Could you check a few things on this drawing? It's one solid part, dimensions in mm from its lowest x, y, z. Coordinates: 2 decimals unless noted, no trailing zeros. Write each loop counter-clockwise with the first axis right and the second up, starting at its lowest first coordinate (ties: lowest second). Pieces come first, ordered by that corner, then holes. Notation, with made-up numbers: (-33.75, 80) - (-19.75, 80) arc R20 ccw to (-19.75, 104) - close; hole circle Ø7 at (22, 41.25). An arc over 180 degrees is marked (long way). Write item = value, one per line. Start each with the question number.
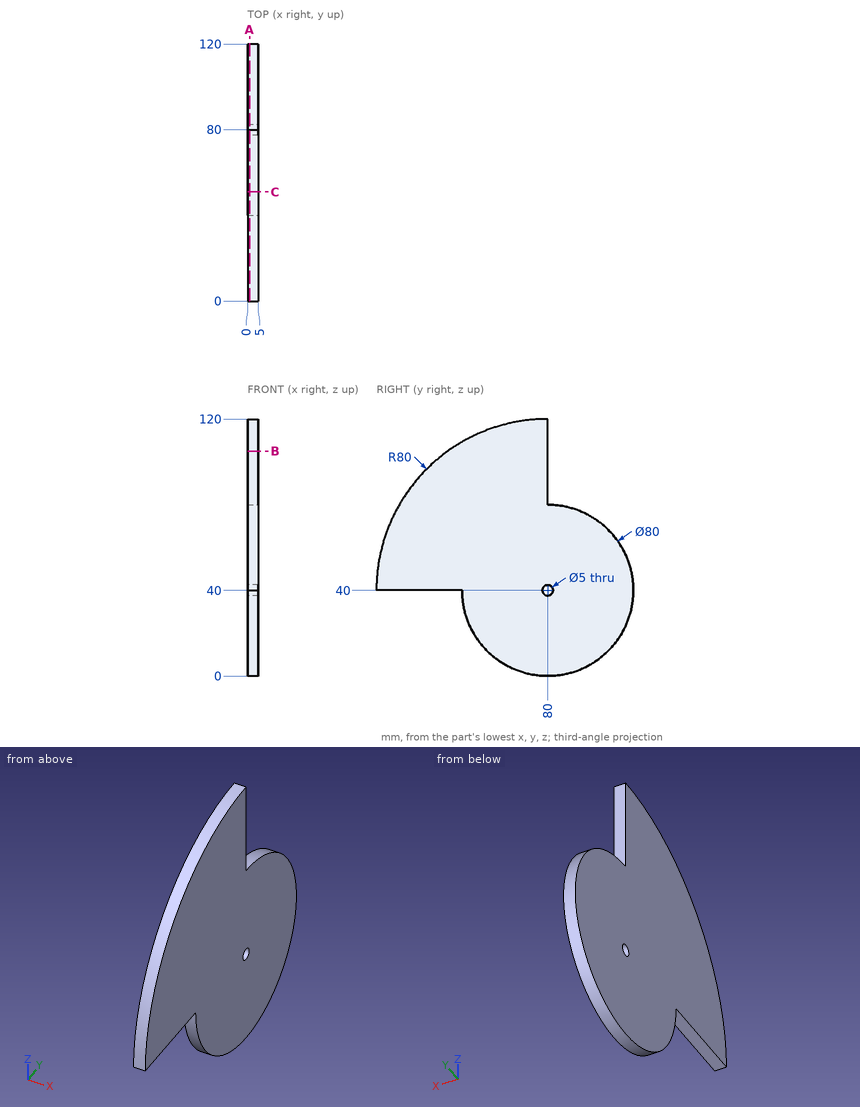
1) Suppose I cut it at B-B on z = 105. Please give me the cut outline in (x, y).
2) Suppose I cut it at A-A on x = 0.9. Please give me the cut outline in (y, z).
3) If I drill on probe 1 along Y at (x, z) = (3.35, 39); probe 2 along Y at (x, z) = (0.35, 28); probe 3 along Y at (x, z) = (3.95, 59.5), over which ranges is the centre line in solid material (lowest first)? Write a range as [from, to].
4) Suppose I cut it at C-C on y = 51. Please give me the cut outline in (x, z), plus the area to 3 significant figures.
5) For P1, Ø1.5, axis at x = 2.5, z = 94.5, coming from the +Y side; P2, Ø1, axis at x = 2.5, y = 107, coming from the -Z side; P3, Ø1.5, axis at x = 3.5, y = 16.5, coming from the -Z side, each with a flat end and sliding along its axis, tell me the tip position at first contact or that it passes through.
Reply:
q1.outline = (0, 33.36) - (5, 33.36) - (5, 80) - (0, 80) - close
q2.outline = (0, 40) - (40, 40) arc R40 ccw (long way) to (80, 80) - (80, 120) arc R80 ccw to start; hole circle Ø5 at (80, 40)
q3.probe_1 = [40.01, 77.71], [82.29, 119.99]
q3.probe_2 = [41.84, 118.16]
q3.probe_3 = [2.41, 114.92]
q4.outline = (0, 12.45) - (5, 12.45) - (5, 114.56) - (0, 114.56) - close
q4.area = 511 mm^2
q5.P1 = 80
q5.P2 = 10.04
q5.P3 = 40
